Geometry: see drawing. Coordinates: mm, zero at the bounding-box minimum. Give positions to 0.01 mm unless a question says otherwise; leave off trailing zeros. Order: outer loops, then holes, each group sorted by start corner. A loop starts at its lowest first (then second) coordinate and runs counter-clockwise, first axis right, second up. Notation, with made-up numbers: (25.5, 1) - (71.5, 1) arc R21 ccw to (71.5, 26) - close; hole circle Ø4 at (15, 28.25). An arc over 180 degrees is marked (long way). Write item = value, one per line. Start each with the question number.
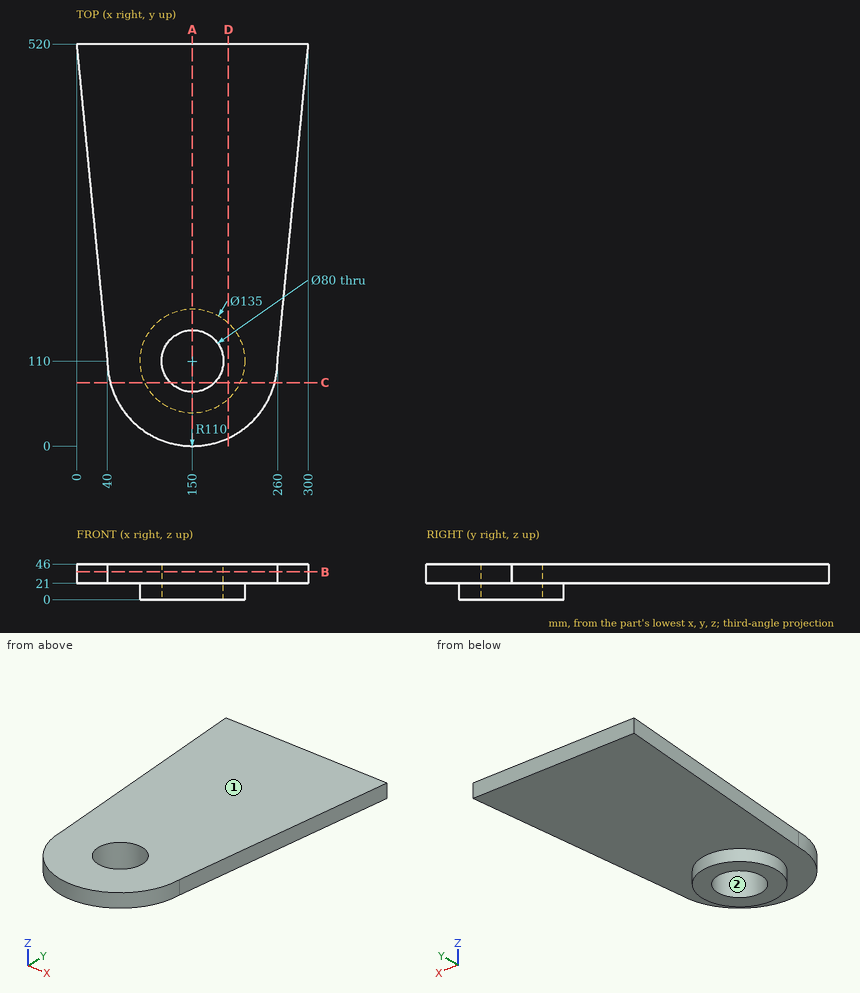
Q1. Contact query for flat-ended pins moving along their axis: pin 1 (1.5 mm diameter, centred on x = 216.5, y = 241.5, fed in from -Z); pin 2 (8 mm diameter, centred on y = 445.5, z = 31, fed in from +X); pin 3 (5 mm diameter, centred on x = 218, z = 31, fed in from -Y). Output: stop coordinate, or through.
Q2. Pull-direction query (Y, two-part tool) for the marked faces 1 and 2; classes: +Y half, -Y half, draft (parallel to the pull), parting line (faces both ways), or undercut.
Q3. Section C-C, the plane y = 82. Return the cut outline in (x, z).
Q4. Section B-B, the plane z = 36. Return the cut outline in (x, y), then the cut area to 3 significant figures.
Q5. Section D-D, the plane x = 196.5. Return the cut outline in (y, z), then the cut area to 3 significant figures.
Q6. Section A-A, the plane x = 150. Return the cut outline in (y, z).
Q7. Material intervals for line 1 along X through (y, z) = (110, 13); line 2 along Y through (x, z) = (150, 26.5); line 3 along X through (y, z) = (110, 36), sorted ascending. Write a range as from..to.
The answers:
q1.pin_1 = 21
q1.pin_2 = 293.12
q1.pin_3 = 21.63
q2.face_1 = draft
q2.face_2 = undercut
q3.outline = (43.62, 21) - (88.58, 21) - (88.58, 0) - (121.43, 0) - (121.43, 46) - (43.62, 46) - close; (178.57, 0) - (211.42, 0) - (211.42, 21) - (256.38, 21) - (256.38, 46) - (178.57, 46) - close
q4.outline = (0, 520) - (40, 110) arc R110 ccw to (260, 110) - (300, 520) - close; hole circle Ø80 at (150, 110)
q4.area = 121,000 mm²
q5.outline = (10.31, 21) - (61.07, 21) - (61.07, 0) - (158.93, 0) - (158.93, 21) - (520, 21) - (520, 46) - (10.31, 46) - close
q5.area = 14,800 mm²
q6.outline = (0, 21) - (42.5, 21) - (42.5, 0) - (70, 0) - (70, 46) - (0, 46) - close; (150, 0) - (177.5, 0) - (177.5, 21) - (520, 21) - (520, 46) - (150, 46) - close
q7.line_1 = 82.5..110, 190..217.5
q7.line_2 = 0..70, 150..520
q7.line_3 = 40..110, 190..260
